Study the drawing (mm; zero at the part's minimum x, y, z) and answer. A direction names the side the tool comes from. Give positions to 0.01 mm unless a question says otherwise; leave off trailing zeros. Loops run counter-clockwise (first coordinate to the right, second up) from the corner with the lowest first, then second, coordinate; pieces in that order, holes last. Notation, with made-up numbers: M 0.25,21 L 22.25,21 A21 ccw 22.25,32 Z; hole C 43.5,48 d1. An arc over 180 degrees is marked long. Return JSON: item names as keys, results as strings.
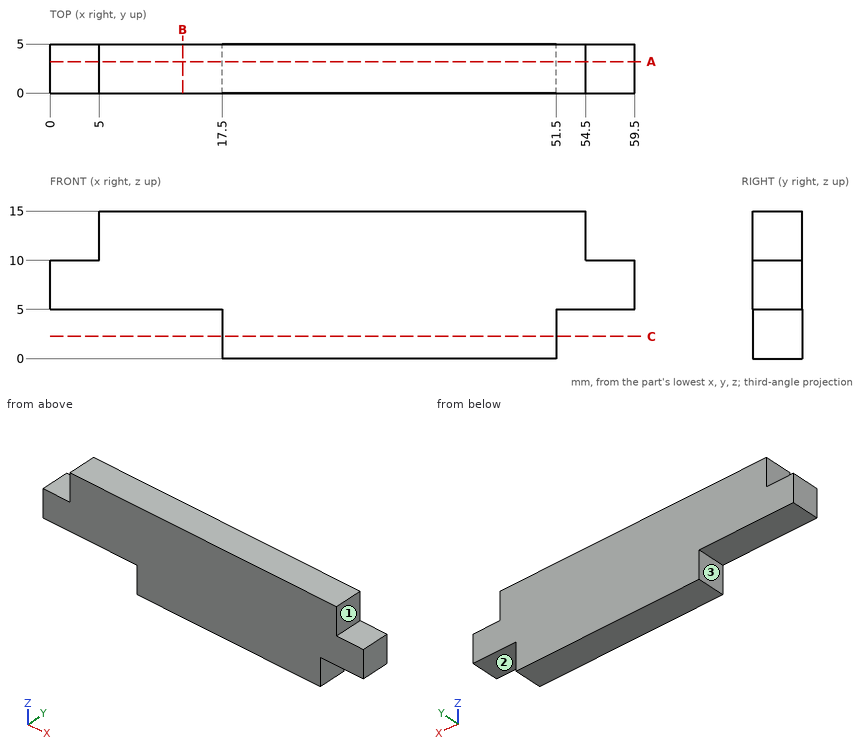
(1) Straight lines are drawn through the part: line 1 along Z through (x, y) = (10.5, 4.25); line 2 along X through (y, z) = (1.95, 10.25); line 3 along X through (y, z) = (2.9, 3.25). For each, find the intervals that lie inside material, in ascending order.
Values follow:
{"line 1": "5 to 15", "line 2": "5 to 54.5", "line 3": "17.5 to 51.5"}
(2) The part is cut by section C-C (z = 2.25). Determine the outline of the cut face in (x, y), and give its area (3 significant figures).
Values follow:
{"outline": "M 17.5,0 L 51.5,0 L 51.5,5 L 17.5,5 Z", "area": "170 mm²"}
(3) A tool of negligible diameter and unlimited length cuts with its end or side. For the marked faces 1, 2 and 3, from which of +Z, -Z, +X, -X, +Y, -Y can it reach the whole face along a straight path? Write none if from no direction.
Values follow:
{"face 1": "+Z, +X, +Y, -Y", "face 2": "-Z, +X, +Y, -Y", "face 3": "-Z, -X, +Y, -Y"}
(4) The part is cut by section B-B (x = 13.5). Determine the outline of the cut face in (y, z).
Values follow:
{"outline": "M 0,5 L 5,5 L 5,15 L 0,15 Z"}
(5) The part is cut by section A-A (y = 3.2). Determine the outline of the cut face in (x, z).
Values follow:
{"outline": "M 0,5 L 17.5,5 L 17.5,0 L 51.5,0 L 51.5,5 L 59.5,5 L 59.5,10 L 54.5,10 L 54.5,15 L 5,15 L 5,10 L 0,10 Z"}
(6) Given pin 1 (4 mm diameter, centred on x = 8.5, z = 7.5, fed in from -Y); pin 2 (1.5 mm diameter, centred on x = 4.5, y = 3, fed in from -Z); pin 3 (1.5 mm diameter, centred on x = 3.5, y = 2, fed in from +Z), each flat-ended and moving along its own axis, determine where each tip first touches the part or whether it passes through.
Values follow:
{"pin 1": "y = 0", "pin 2": "z = 5", "pin 3": "z = 10"}
